Autodesk Inventor part; units mm, degrees
ref_plane "YZ Plane" through (0, 0, 0) normal (1, 0, 0) x (0, 1, 0)
ref_plane "XZ Plane" through (0, 0, 0) normal (0, 1, 0) x (-1, 0, 0)
ref_plane "XY Plane" through (0, 0, 0) normal (0, 0, 1) x (1, 0, 0)
sketch "Sketch1" plane through (0, 0, 0) normal (1, 0, 0) x (0, 1, 0)
  line L0 (0, 0) -> (45.2437, 0)
  line L1 (45.2437, 0) -> (45.2438, -57.15)
  line L2 (45.2438, -57.15) -> (0, -57.15)
  line L3 (0, -57.15) -> (0, 0)
  dimension "d0" = 45.2437
  dimension "d1" = 57.15
extrude "Extrusion1" add sketch "Sketch1" along normal blind 4.7625
sketch "Sketch3" plane through (4.7625, 0, 0) normal (1, 0, 0) x (0, 0, -1)
  line L0 (0, 45.2437) -> (0, 0)
  line L1 (0, 0) -> (57.15, 0)
  line L2 (57.15, 0) -> (57.15, 45.2438)
  line L3 (57.15, 45.2438) -> (0, 45.2437)
  line L4 (0, 0) -> (25.4, 0)
  line L5 (25.4, 0) -> (25.4, 4.7625)
  line L6 (25.4, 4.7625) -> (0, 4.7625)
  line L7 (0, 4.7625) -> (0, 0)
  dimension "d8" = 4.7625
extrude "Extrusion3" add sketch "Sketch3" along normal blind 19.05 contours L6 L5 L1 L0
sketch "Sketch4" plane through (0, 0, 0) normal (-1, 0, 0) x (0, 0, 1)
  line L0 (0, 0) -> (0, 45.2437)
  line L1 (0, 45.2437) -> (-57.15, 45.2438)
  line L2 (-57.15, 45.2438) -> (-57.15, 0)
  line L3 (-57.15, 0) -> (0, 0)
  line L4 (-57.15, 45.2438) -> (0, 45.2437)
  line L5 (-57.15, 45.2438) -> (-44.45, 45.2438)
  line L6 (-57.15, 29.3688) -> (-57.15, 45.2438)
  line L7 (-57.15, 0) -> (-57.15, 45.2438)
  line L8 (-57.15, 32.5438) -> (-44.45, 32.5438)
  line L9 (-44.45, 32.5438) -> (-44.45, 16.6688)
  line L10 (-44.45, 16.6688) -> (-57.15, 16.6688)
  line L11 (-57.15, 16.6688) -> (-57.15, 32.5438)
  point P0 (-12.7, 45.2437)
  dimension "d48" = 15.875
  dimension "d49" = 12.7
  dimension "d50" = 12.7
extrude "Extrusion4" add sketch "Sketch4" along normal blind 7.9375 contours L2 L8 L9 L10
sketch "Sketch5" plane through (4.7625, 0, 0) normal (1, 0, 0) x (0, 0, -1)
  line L0 (25.4, 4.7625) -> (25.4, 0)
  line L1 (25.4, 0) -> (57.15, 0)
  line L2 (57.15, 0) -> (57.15, 45.2438)
  line L3 (57.15, 45.2438) -> (0, 45.2437)
  line L4 (0, 45.2437) -> (0, 4.7625)
  line L5 (0, 4.7625) -> (25.4, 4.7625)
  line L6 (0, 45.2437) -> (0, 40.4812)
  line L7 (0, 40.4812) -> (12.7, 40.4812)
  line L8 (12.7, 40.4812) -> (12.7, 45.2437)
  line L9 (12.7, 45.2437) -> (0, 45.2437)
  point P0 (0, 0)
  point P1 (50.8, 24.6063)
  dimension "d16" = 20.6375
  dimension "d17" = 6.35
hole "Hole1" at (4.7625, 24.6063, -50.8) direction (-1, 0, 0) diameter 3.683 depth 14.9352 tip angle 118
sketch "Sketch6" plane through (4.7625, 4.7625, 0) normal (0, 1, 0) x (1, 0, 0)
  line L0 (0, 0) -> (0, 25.4)
  line L1 (0, 0) -> (19.05, 0)
  line L2 (19.05, 25.4) -> (19.05, 0)
  line L3 (0, 25.4) -> (19.05, 25.4)
  point P0 (-4.7625, 0)
  point P1 (9.525, 9.525)
  dimension "d25" = 9.525
  dimension "d26" = 9.525
hole "Hole2" at (14.2875, 4.7625, -9.525) direction (0, -1, 0) diameter 12.7 depth 3.175
sketch "Sketch10" plane through (0, 45.2438, 0) normal (0, 1, 0) x (1, 0, 0)
  line L0 (0, 0) -> (0, 57.15)
  line L1 (0, 0) -> (4.7625, 0)
  line L2 (4.7625, 57.15) -> (4.7625, 0)
  line L3 (0, 57.15) -> (4.7625, 57.15)
  point P0 (0, 0)
  point P1 (11.1125, 6.35)
hole "Hole3" at (11.1125, 45.2438, -6.35) direction (0, -1, 0) diameter 2.6416 depth 10.9728 tip angle 118
sketch "Sketch11" plane through (0, 0, -57.15) normal (0, -1, 0) x (1, 0, 0)
  line L0 (0, 0) -> (0, 57.15)
  line L1 (0, 0) -> (4.7625, 0)
  line L2 (4.7625, 31.75) -> (4.7625, 0)
  line L3 (4.7625, 31.75) -> (23.8125, 31.75)
  line L4 (23.8125, 57.15) -> (23.8125, 31.75)
  line L5 (0, 57.15) -> (23.8125, 57.15)
  point P0 (15.0812, 38.1)
  dimension "d58" = 6.35
hole "Hole4" at (15.0812, 0, -19.05) direction (0, 1, 0) diameter 2.6416 end through all
sketch "Sketch12" plane through (4.7625, 0, 0) normal (1, 0, 0) x (0, 0, -1)
  circle A0 centre (50.8, 24.6063) radius 1.8415
  line L0 (25.4, 4.7625) -> (25.4, 0)
  line L1 (25.4, 0) -> (57.15, 0)
  line L2 (57.15, 0) -> (57.15, 45.2438)
  line L3 (57.15, 45.2438) -> (0, 45.2437)
  line L4 (0, 45.2437) -> (0, 4.7625)
  line L5 (0, 4.7625) -> (25.4, 4.7625)
  point P0 (0, 0)
  point P1 (50.8, 10.3124)
  point P2 (30.7975, 6.5024)
  dimension "d66" = 6.35
  dimension "d67" = 10.3124
  dimension "d68" = 6.5024
  dimension "d69" = 26.3525
hole "Hole5" at (4.7625, 10.3124, -50.8) at (4.7625, 6.5024, -30.7975) direction (-1, 0, 0) diameter 3.556 end through all
sketch "Sketch13" plane through (4.7625, 0, 0) normal (1, 0, 0) x (0, 0, -1)
  line L0 (0, 45.2437) -> (0, 4.7625)
  point P0 (0, 0)
  point P1 (5.08, 42.0254)
  point P2 (20.32, 42.0254)
  dimension "d77" = 5.08
  dimension "d78" = 15.24
hole "Hole6" at (4.7625, 42.0254, -5.08) at (4.7625, 42.0254, -20.32) direction (-1, 0, 0) diameter 2.6416 end through all
properties part number "WheelIntake4.0Base"
Geometry: final body of the model. Coordinates: model frame, mm. A direction names the side the tool comes from. Coordinates: 2 decimals unless noted, no trailing zeros. Order: outer loops, then holes, each group sorted by start corner. A loop starts at its lowest first (then second) coordinate and runs counter-clockwise, first axis right, second up. Notation, with made-up numbers: (23.25, 30.25) - (40.25, 30.25) arc R20 ccw to (40.25, 34.25) - close; hole circle Ø2 at (30, 7). An arc over 180 degrees is marked (long way). Write each question's results on one line, items separated by ' | '.
(1) Section query B-B, the plane y = 4. Count the separate pieces of the cut face and the enclosed holes in it, plus the area to 3 significant figures.
Values found:
separate pieces: 1 | enclosed holes: 2 | area: 624 mm²
(2) Section query A-A, the plane z = -51. Return the cut outline in (x, y), plus the area to 3 significant figures.
Values found:
outline: (-7.94, 16.67) - (0, 16.67) - (0, 12.08) - (4.76, 12.08) - (4.76, 22.78) - (-7.94, 22.78) - close; (-7.94, 26.44) - (4.76, 26.44) - (4.76, 45.24) - (0, 45.24) - (0, 32.54) - (-7.94, 32.54) - close; (0, 0) - (4.76, 0) - (4.76, 8.55) - (0, 8.55) - close | area: 278 mm²
(3) First-contact query: pin 1 Ø2 at (y, z) = (28.5, -24.5) entering from -X; pin 2 Ø4 at (y, z) = (6.5, -30.8) entering from +X; pin 3 Ø2.5 at (x, z) = (-4, -48.5) entering from -Y. Flat tips, straight axial feed; report the tip coordinate or a pass-through.
Values found:
pin 1: stops at x = 0 | pin 2: stops at x = 4.76 | pin 3: stops at y = 16.67
(4) Section query D-D, the plane x = 22.5. Return the cut outline in (y, z).
Values found:
outline: (0, -25.4) - (4.76, -25.4) - (4.76, 0) - (0, 0) - close
(5) Set-up query: faces 1 (the face through (-4, 16.669, -51)), 2 (the face through (14, 1.588, -10)), 3 (the face through (-4, 32.544, -51)). Return all of +Z, -Z, +X, -X, +Y, -Y with unobstructed straight access to the full face (end or side cutting, diameter ignored); none if empty.
Values found:
face 1: +Z, -Z, -X, -Y | face 2: +Y | face 3: +Z, -Z, -X, +Y
(6) Line query: line 1 (Y direction, x = 2, z = -50.8); line 2 (Y direction, x = 3, z = -5.08); line 3 (X direction, y = 22, z = -15.5). Output: solid intervals per line, ascending. Write a range as [from, to].
Values found:
line 1: y = [0, 8.53], [12.09, 22.76], [26.45, 45.24] | line 2: y = [0, 40.7], [43.35, 45.24] | line 3: x = [0, 4.76]
(7) Section query C-C, the plane z = -5.08. Return the cut outline in (x, y), plus the area to 3 significant figures.
Values found:
outline: (0, 0) - (23.81, 0) - (23.81, 4.76) - (18.82, 4.76) - (18.82, 1.59) - (9.75, 1.59) - (9.75, 4.76) - (4.76, 4.76) - (4.76, 40.7) - (0, 40.7) - close; (0, 43.35) - (4.76, 43.35) - (4.76, 45.24) - (0, 45.24) - close | area: 265 mm²
(8) Mould query, pull axis Y, two halves, no side actions, for faces 4 (the face through (14, 2, -25.4)), 5 (the face through (12, 4.762, -16)), 6 (the face through (2.35, 6.42, -29.02)). Classes: +Y half, -Y half, draft (parallel to the pull), parting line (faces both ways), or undercut.
Values found:
face 4: draft | face 5: +Y half | face 6: undercut
